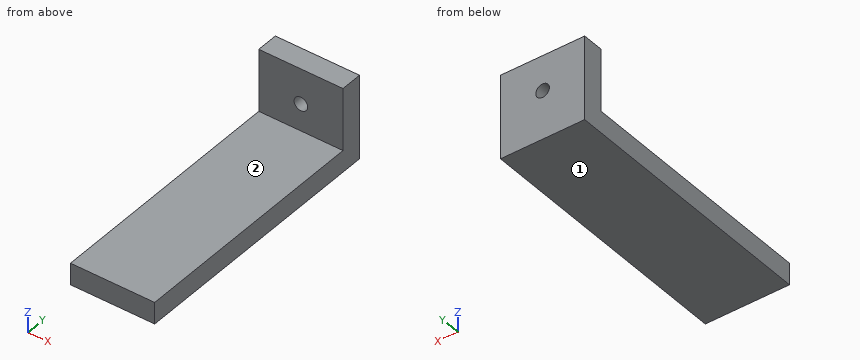
from build123d import *

# Parameters (mm, degrees)
F1_DEPTH = 19.685
F3_D     = 3.175


with BuildPart() as f1:
    # F0 (on Right) → F1 (new body)
    with BuildSketch(Plane.YZ):
        Polygon((-35.253628, -10.520633), (-35.253628, -15.600633), (27.738372, -15.600633), (27.738372, 4.084367), (22.658372, 4.084367), (22.658372, -10.520633), align=None)
    extrude(amount=F1_DEPTH)

    # F3 (through all)
    with Locations(Plane(origin=(0, 27.738372, 0), x_dir=(-1, 0, 0), z_dir=(0, 1, 0))):
        with Locations((-9.8425, -4.170633)):
            Hole(F3_D / 2)


solid = f1.part
Work out the finished part from the listing and answer in its coordinate system (mm). Face numbers are marked on the shaded views. A direction names the side the tool comes from. Round coordinates to 2 decimals unless told otherwise and drop trailing zeros. Write each loop counter-clockwise with the first axis right and the second up, starting at its lowest first coordinate (ties: lowest second). Pieces come first, ordered by that corner, then holes.
1) A tool of negligible diameter and unlimited length cuts with its end or side. For the marked faces 1 and 2, from which of +Z, -Z, +X, -X, +Y, -Y can it reach the whole face along a straight path? Write none if from no direction.
2) A cutting plane is placed at B-B (y = 20.5). Give the vertices of the cut face in (x, z) (3 decimals).
3) A cutting plane is placed at C-C (z = -7.5). Give the vertices of the cut face in (x, y) (3 decimals).
4) A cutting plane is placed at A-A (x = 7.5). Give the vertices of the cut face in (y, z), plus the area to 3 significant figures.
5) Given pin 1 Ø1 at (x, z) = (6.5, -7.5) entering from -Y; pin 2 Ø6 at (x, y) = (8, -15) entering from +Z, each flat-ended and moving along its own axis, determine where each tip first touches the part or whether it passes through.
6) Straight lines are drawn through the part: line 1 (Z direction, x = 6.5, y = -10); line 2 (Y direction, x = 5.75, z = 1); line 3 (X direction, y = 25, z = -2.75) (3 decimals). For each, find the intervals that lie inside material, in ascending order.
Completed:
1. face 1: -Z, +X, -X, +Y, -Y
1. face 2: +Z, +X, -X, -Y
2. outline: (0, -15.601) - (19.685, -15.601) - (19.685, -10.521) - (0, -10.521) - close
3. outline: (0, 22.658) - (19.685, 22.658) - (19.685, 27.738) - (0, 27.738) - close
4. outline: (-35.25, -15.6) - (27.74, -15.6) - (27.74, 4.08) - (22.66, 4.08) - (22.66, -10.52) - (-35.25, -10.52) - close
4. area: 394 mm2
5. pin 1: stops at y = 22.66
5. pin 2: stops at z = -10.52
6. line 1: z = -15.6 to -10.52
6. line 2: y = 22.66 to 27.74
6. line 3: x = 0 to 9.134, 10.551 to 19.685
